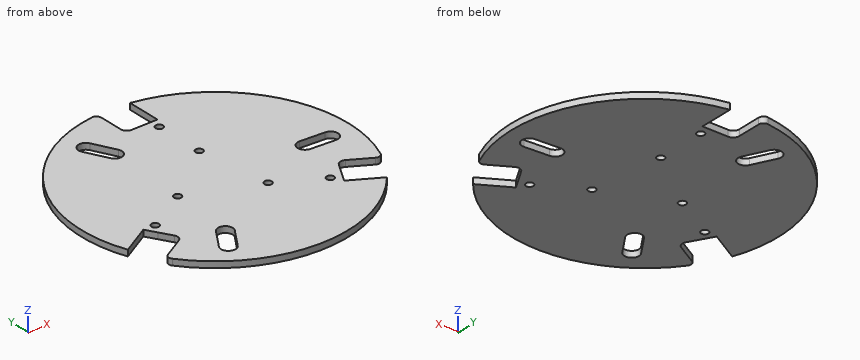
from build123d import *

# Parameters (mm, degrees)
SKETCH1_R           = 1.905
BOSS_EXTRUDE1_DEPTH = 3.175
FILLET1_R           = 2.54


with BuildPart() as part:
    # Sketch1 → Boss-Extrude1 (new body)
    with BuildSketch(Plane.XY):
        with BuildLine():
            Line((-64.912044694, -24.170240567), (-49.756080512, -15.419940567))
            Line((-49.756080512, -15.419940567), (-46.581080512, -20.919201881))
            Line((-46.581080512, -20.919201881), (-43.088580512, -26.968389327))
            ThreePointArc((-43.088580512, -26.968389327), (-42.771396671, -29.377639795), (-44.250711169, -31.305519984))
            Line((-44.250711169, -31.305519984), (-57.337460999, -38.861158521))
            ThreePointArc((-57.337460999, -38.861158521), (-3.292499409, -69.187668866), (53.388064694, -44.130359433))
            Line((53.388064694, -44.130359433), (38.232100512, -35.380059433))
            Line((38.232100512, -35.380059433), (41.407100512, -29.880798119))
            Line((41.407100512, -29.880798119), (44.899600512, -23.831610673))
            ThreePointArc((44.899600512, -23.831610673), (46.827480701, -22.352296175), (49.236731169, -22.669480016))
            Line((49.236731169, -22.669480016), (62.323480999, -30.225118553))
            ThreePointArc((62.323480999, -30.225118553), (61.564528571, 31.742446303), (11.52398, 68.3006))
            Line((11.52398, 68.3006), (11.52398, 50.8))
            Line((11.52398, 50.8), (5.17398, 50.8))
            Line((5.17398, 50.8), (-1.81102, 50.8))
            ThreePointArc((-1.81102, 50.8), (-4.05608403, 51.72993597), (-4.98602, 53.975))
            Line((-4.98602, 53.975), (-4.98602, 69.086277074))
            ThreePointArc((-4.98602, 69.086277074), (-58.272029162, 37.445222563), (-64.912044694, -24.170240567))
        make_face()
        with Locations((-43.769171461, -15.629571224)):
            Circle(SKETCH1_R, mode=Mode.SUBTRACT)
        with Locations((-21.772126205, -2.929571224)):
            Circle(SKETCH1_R, mode=Mode.SUBTRACT)
        with Locations((13.423146205, -17.390428776)):
            Circle(SKETCH1_R, mode=Mode.SUBTRACT)
        with Locations((35.420191461, -30.090428776)):
            Circle(SKETCH1_R, mode=Mode.SUBTRACT)
        with Locations((8.34898, 45.72)):
            Circle(SKETCH1_R, mode=Mode.SUBTRACT)
        with Locations((8.34898, 20.32)):
            Circle(SKETCH1_R, mode=Mode.SUBTRACT)
        with BuildLine():
            Line((-21.860648036, 52.941011205), (-16.243380607, 41.550826544))
            ThreePointArc((-16.243380607, 41.550826544), (-17.975255776, 36.448590916), (-23.077491403, 38.180466086))
            Line((-23.077491403, 38.180466086), (-28.694758833, 49.570650747))
            ThreePointArc((-28.694758833, 49.570650747), (-26.962883664, 54.672886375), (-21.860648036, 52.941011205))
        make_face(mode=Mode.SUBTRACT)
        with BuildLine():
            Line((56.778584624, -7.53862906), (44.105761638, -6.708233023))
            ThreePointArc((44.105761638, -6.708233023), (40.553033554, -2.657267317), (44.60399926, 0.895460768))
            Line((44.60399926, 0.895460768), (57.276822246, 0.065064732))
            ThreePointArc((57.276822246, 0.065064732), (60.829550331, -3.985900975), (56.778584624, -7.53862906))
        make_face(mode=Mode.SUBTRACT)
        with BuildLine():
            Line((-34.917936587, -45.402382145), (-27.862381032, -34.84259352))
            ThreePointArc((-27.862381032, -34.84259352), (-22.577777778, -33.7913236), (-21.526507857, -39.075926854))
            Line((-21.526507857, -39.075926854), (-28.582063413, -49.635715479))
            ThreePointArc((-28.582063413, -49.635715479), (-33.866666667, -50.686985399), (-34.917936587, -45.402382145))
        make_face(mode=Mode.SUBTRACT)
    extrude(amount=BOSS_EXTRUDE1_DEPTH)

    # Fillet1
    fillet1_edges = [part.edges().sort_by_distance(p)[0] for p in [
        (-4.98602, 69.086277074, 1.5875),
        (62.323480999, -30.225118553, 1.5875),
        (-57.337460999, -38.861158521, 1.5875),
    ]]
    fillet(fillet1_edges, radius=FILLET1_R)


solid = part.part
Verification items for the finished model (mm, model axes). Give positions to 0.01 mm unless a question says otherwise; leave off trailing zeros. Write each loop counter-clockwise with the first axis right and the second up, starting at its lowest first coordinate (ties: lowest second). Pieces come first, ordered by that corner, then holes. Notation, with made-up numbers: M 32.5,63.25 L 54.5,63.25 A24 ccw 54.5,88.25 Z; hole C -5,3.25 d8. An arc over 180 degrees is marked long. Put each result on its own line as item: value. Start each with the question number.
1. Section check D-D (z = 1.45). Give the number of separate pieces and of enclosed holes in the cut face, and give its area (3 significant figures).
2. Go/stop test with flat-tipped pins: pin 1 Ø3.5 at (x, y) = (-21.77, -2.93) entering from -Z; pin 2 Ø1 at (y, z) = (63.5, 2) entering from -X; pin 3 Ø1 at (y, z) = (63, 2) entering from +X; pin 4 Ø1 at (x, z) = (3.5, 1.5) entering from +Y. Record where each tip stops, or that it passes through.
3. Section check A-A (y = 45.72). Record the cut outline in (x, z) (3 decimals), and give its area (3 significant figures).
4. Scan lines: line 1 along X through (y, z) = (-4.5, 2.35); line 2 along Y through (x, z) = (-24, 1.7); line 3 along Y through (x, z) = (54.5, 1.6). Record each from-to range of solid material in increasing order. Write a range as [from, to].
5. Section check B-B (y = 20.32). Record the cut outline in (x, z) (3 decimals).
6. Section check C-C (x = -31.75). Record the cut outline in (y, z) (3 decimals), and give its area (3 significant figures).
Answer list:
1. separate pieces: 1
1. enclosed holes: 9
1. area: 13,700 mm2
2. pin 1: through
2. pin 2: x = -28.79
2. pin 3: x = 29.86
2. pin 4: y = 50.8
3. outline: M -52.033,0 L -26.796,0 L -26.796,3.175 L -52.033,3.175 Z; M -18.299,0 L 6.444,0 L 6.444,3.175 L -18.299,3.175 Z; M 10.254,0 L 52.033,0 L 52.033,3.175 L 10.254,3.175 Z
3. area: 291 mm2
4. line 1: [-69.12, -22.85], [-20.69, 40.89], [60.76, 69.12]
4. line 2: [-64.98, -42.78], [-33.21, 40.05], [54.85, 64.98]
4. line 3: [-25.71, -7.39], [0.25, 42.75]
5. outline: M -66.218,0 L 6.444,0 L 6.444,3.175 L -66.218,3.175 Z; M 10.254,0 L 66.218,0 L 66.218,3.175 L 10.254,3.175 Z
6. outline: M -61.561,0 L -51.329,0 L -51.329,3.175 L -61.561,3.175 Z; M -40.661,0 L 61.561,0 L 61.561,3.175 L -40.661,3.175 Z
6. area: 357 mm2
